Read the model definition and answer for the solid it produces. Units are mm, in the model's axes. A direction names the side the tool comes from. Round coordinates to 2 decimals unless told otherwise and drop trailing zeros. Order: outer loops, then holes, each group sorted by start corner. A loop starts at its lowest first (then second) coordinate and runs counter-clockwise, first axis right, second up. Notation, with made-up numbers: (-12, 55.5) -> (-8, 55.5) arc R17 ccw to (-8, 59.5) -> close; hole circle Ø3 at (11.5, 89.5). An arc over 180 degrees is marked (long way). Use a Markdown table: item, result. Add a question column.
1. Consider L1, parallel to X at y = 30, z = 3; L2, parallel to Y at x = -17.5, z = 4.75; L3, parallel to Y at x = 22, z = 0.75. Determine where each line is inside the solid, lowest interval first. Write a range as [from, to].
2. Section C-C, the plane y = -29 is taken. Give the vertices of the cut face in (x, z), then the cut area to 3 significant figures.
3. Given pin 1 (1.5 mm diameter, centred on x = -41.5, z = 5, fed in from -Y); pin 2 (1.9 mm diameter, centred on y = 84, z = 4.5, fed in from +X); pin 3 (1.5 mm diameter, centred on y = -11.5, z = 1.5, fed in from +X), each flat-ended and moving along its own axis, determine where each tip first touches the part or whether it passes through.
4. For faces 4 (the face through (0.94, 102.84, 3.13)), 5 (the face through (0.062, 8.746, 3.131)), determine the directions among +Z, -Z, +X, -X, +Y, -Y from which every point of the face is accessible in a straight line to the end or side of a thin tool.
5. Section B-B, the plane y = -55.5 is taken. Give the vertices of the cut face in (x, z).
6. Section D-D, the plane z = 3.75 is taken. Give the number of separate pieces and of enclosed holes in the cut face, then the cut area to 3 significant figures.
7. The mould has two halves that part along X. Classify faces 1 (the face through (22.863, 33.17, 3.219)), 2 (the face through (15, 19, 6.35)), 3 (the face through (-1.48, -66.11, 3.13)): +X half, -X half, draft (parallel to the pull), parting line (faces both ways), or undercut.
8. Section A-A, the plane x = 0 is taken. Give the vertices of the cut face in (y, z).
```python
from build123d import *

# Parameters (mm, degrees)
BOSS_EXTRUDE1_DEPTH = 6.35
CUT_EXTRUDE1_REACH  = 8.35
SKETCH2_W           = 29.21
SKETCH2_H           = 29.21
FILLET1_R           = 5.08
BOSS_EXTRUDE2_DEPTH = 6.35
FILLET2_R           = 5.08


with BuildPart() as part:
    # Sketch1 → Boss-Extrude1 (new body)
    with BuildSketch(Plane.XY):
        with BuildLine():
            ThreePointArc((-54.695205109, 69.85), (-67.085998682, 35.772421109), (-69.83842006, -0.383315988))
            ThreePointArc((-69.83842006, -0.383315988), (0, -66.125848112), (69.83842006, -0.383315988))
            ThreePointArc((69.83842006, -0.383315988), (67.085998682, 35.772421109), (54.695205109, 69.85))
            ThreePointArc((54.695205109, 69.85), (0, 102.847096123), (-54.695205109, 69.85))
        make_face()
        with BuildLine():
            Line((-50.8, 63.5), (50.8, 63.5))
            ThreePointArc((50.8, 63.5), (61.265344619, 32.573068924), (63.5, 0))
            ThreePointArc((63.5, 0), (0, -59.775848112), (-63.5, 0))
            ThreePointArc((-63.5, 0), (-61.265344619, 32.573068924), (-50.8, 63.5))
        make_face(mode=Mode.SUBTRACT)
    extrude(amount=BOSS_EXTRUDE1_DEPTH)

    # Sketch2 → Cut-Extrude1 (cut, up to next)
    with BuildSketch(Plane.XY.offset(6.35), mode=Mode.PRIVATE) as cut_extrude1_sk1:
        with Locations((0, 83.173548061)):
            Rectangle(SKETCH2_W, SKETCH2_H)
    cut_extrude1_tool1 = extrude(cut_extrude1_sk1.sketch, amount=-CUT_EXTRUDE1_REACH, mode=Mode.PRIVATE) & part.part
    add(cut_extrude1_tool1.solids().sort_by_distance((0, 83.173548, 6.35))[0], mode=Mode.SUBTRACT)

    # Fillet1
    fillet1_edges = [part.edges().sort_by_distance(p)[0] for p in [
        (14.605, 97.778548061, 3.175),
        (14.605, 68.568548061, 3.175),
        (-14.605, 68.568548061, 3.175),
        (-14.605, 97.778548061, 3.175),
    ]]
    fillet(fillet1_edges, radius=FILLET1_R)

    # Sketch3 → Boss-Extrude2 (add)
    with BuildSketch(Plane.XY.offset(6.35)):
        with BuildLine():
            Line((48.313199114, 63.5), (0, 5.922571386))
            Line((0, 5.922571386), (2.486800886, 2.958917496))
            Line((2.486800886, 2.958917496), (51.704078268, 61.613784634))
            ThreePointArc((51.704078268, 61.613784634), (51.255922445, 62.55875362), (50.8, 63.5))
            Line((50.8, 63.5), (48.313199114, 63.5))
        make_face()
        with BuildLine():
            Line((-48.313199114, 63.5), (-50.8, 63.5))
            ThreePointArc((-50.8, 63.5), (-51.255922445, 62.55875362), (-51.704078268, 61.613784634))
            Line((-51.704078268, 61.613784634), (-2.486800886, 2.958917496))
            Line((-2.486800886, 2.958917496), (0, 5.922571386))
            Line((0, 5.922571386), (-48.313199114, 63.5))
        make_face()
        Polygon((0, 5.922571386), (-2.486800886, 2.958917496), (0, -0.004736394), (2.486800886, 2.958917496), align=None)
        with BuildLine():
            Line((2.486800886, 2.958917496), (0, -0.004736394))
            Line((0, -0.004736394), (38.967470095, -46.444358875))
            ThreePointArc((38.967470095, -46.444358875), (40.455837743, -45.254867888), (41.907916796, -44.021339013))
            Line((41.907916796, -44.021339013), (2.486800886, 2.958917496))
        make_face()
        with BuildLine():
            Line((0, -0.004736394), (-2.486800886, 2.958917496))
            Line((-2.486800886, 2.958917496), (-41.907916796, -44.021339013))
            ThreePointArc((-41.907916796, -44.021339013), (-40.455837743, -45.254867888), (-38.967470095, -46.444358875))
            Line((-38.967470095, -46.444358875), (0, -0.004736394))
        make_face()
    extrude(amount=-BOSS_EXTRUDE2_DEPTH)

    # Fillet2
    fillet2_edges = [part.edges().sort_by_distance(p)[0] for p in [
        (48.313199114, 63.5, 3.175),
        (0, 5.922571386, 3.175),
        (-48.313199114, 63.5, 3.175),
        (-51.704078268, 61.613784634, 3.175),
        (-2.486800886, 2.958917496, 3.175),
        (-41.907916796, -44.021339013, 3.175),
        (-38.967470095, -46.444358875, 3.175),
        (0, -0.004736394, 3.175),
        (38.967470095, -46.444358875, 3.175),
        (41.907916796, -44.021339013, 3.175),
        (2.486800886, 2.958917496, 3.175),
        (51.704078268, 61.613784634, 3.175),
    ]]
    fillet(fillet2_edges, radius=FILLET2_R)


solid = part.part
```
Verdict:
| question | item | result |
|---|---|---|
| 1 | L1 | x = [-68.2, -61.75], [-25.18, -20.2], [20.2, 25.18], [61.75, 68.2] |
| 1 | L2 | y = [-63.9, -57.32], [-20.86, -14.93], [20.85, 26.78], [63.5, 100.32] |
| 1 | L3 | y = [-62.58, -55.85], [-26.22, -20.3], [26.21, 32.14], [63.5, 98.8] |
| 2 | outline | (-61.78, 0) -> (-54.48, 0) -> (-54.48, 6.35) -> (-61.78, 6.35) -> close; (-29.3, 0) -> (-24.33, 0) -> (-24.33, 6.35) -> (-29.3, 6.35) -> close; (24.33, 0) -> (29.3, 0) -> (29.3, 6.35) -> (24.33, 6.35) -> close; (54.48, 0) -> (61.78, 0) -> (61.78, 6.35) -> (54.48, 6.35) -> close |
| 2 | area | 156 mm2 |
| 3 | pin 1 | stops at y = -53.03 |
| 3 | pin 2 | stops at x = 45.34 |
| 3 | pin 3 | stops at x = 68.43 |
| 4 | face 4 | +Z, -Z, +Y |
| 4 | face 5 | +Z, -Z |
| 5 | outline | (-37.07, 0) -> (-22.93, 0) -> (-22.93, 6.35) -> (-37.07, 6.35) -> close; (22.93, 0) -> (37.07, 0) -> (37.07, 6.35) -> (22.93, 6.35) -> close |
| 6 | separate pieces | 1 |
| 6 | enclosed holes | 5 |
| 6 | area | 5,770 mm2 |
| 7 | face 1 | undercut |
| 7 | face 2 | draft |
| 7 | face 3 | parting line |
| 8 | outline | (-66.13, 0) -> (-59.78, 0) -> (-59.78, 6.35) -> (-66.13, 6.35) -> close; (-2.83, 0) -> (8.75, 0) -> (8.75, 6.35) -> (-2.83, 6.35) -> close; (63.5, 0) -> (68.57, 0) -> (68.57, 6.35) -> (63.5, 6.35) -> close; (97.78, 0) -> (102.85, 0) -> (102.85, 6.35) -> (97.78, 6.35) -> close |
